Build history of the part. All positions in model axes, mm. A direction names the side the tool comes from. Round coordinates to 2 decimals unless told otherwise and drop trailing zeros. Write each loop counter-clockwise with the first axis right and the second up, starting at its lowest first coordinate (ties: lowest second). Pieces come first, ordered by that corner, then holes. Notation, with made-up numbers: M 57.25,-13.75 L 65.25,-13.75 A7 ccw 65.25,-0.75 Z; hole C -13.5,73 d8. An arc over 180 degrees is marked long. Use a Markdown table: item, result.
from build123d import *

# Parameters (mm, degrees)
SZKIC1_W                    = 115
SZKIC1_H                    = 56
DODANIE_WYCI_GNI_CIE1_DEPTH = 33
SZKIC2_R                    = 5.5
DODANIE_WYCI_GNI_CIE2_DEPTH = 22
DODANIE_WYCI_GNI_CIE3_DEPTH = 15


with BuildPart() as part:
    # Szkic1 → Dodanie-wyciągnięcie1 (new body)
    with BuildSketch(Plane(origin=(0, 0, 0), x_dir=(1, 0, 0), z_dir=(0, 1, 0))):
        with Locations((57.5, 28)):
            Rectangle(SZKIC1_W, SZKIC1_H)
    extrude(amount=DODANIE_WYCI_GNI_CIE1_DEPTH)

    # Szkic2 → Dodanie-wyciągnięcie2 (add)
    with BuildSketch(Plane(origin=(115, 0, 0), x_dir=(0, 0, -1), z_dir=(1, 0, 0))):
        with Locations((28, 16.5)):
            Circle(SZKIC2_R)
    extrude(amount=DODANIE_WYCI_GNI_CIE2_DEPTH)

    # Szkic3 → Dodanie-wyciągnięcie3 (add)
    with BuildSketch(Plane.ZY):
        Polygon((-34, 16.5), (-34, 12), (-22, 12), (-22, 16.5), (-22, 21), (-34, 21), align=None)
    extrude(amount=DODANIE_WYCI_GNI_CIE3_DEPTH)


solid = part.part
Q1. Cut at A-A on y = 16.5. Give the cut face in (x, z), and give its area (3 significant figures).
Response values:
| item | result |
|---|---|
| outline | M -15,-34 L 0,-34 L 0,-56 L 115,-56 L 115,-33.5 L 137,-33.5 L 137,-22.5 L 115,-22.5 L 115,0 L 0,0 L 0,-22 L -15,-22 Z |
| area | 6,860 mm2 |
Q2. Which spindle directions (+Z, -Z, +X, -X, +Y, -Y) get a long thin tool onto all of the face, cutting with end or side? Do faces 1 (the cylindrical face through (125.8, 13.2, -23.6)), 2 (the flat face through (-7, 21, -28)), 3 (the flat face through (-7, 17, -34)), 4 (the flat face through (-7, 12, -28)), 5 (the flat face through (-7, 16, -22)). Say none if no direction does.
Response values:
| item | result |
|---|---|
| face 1 | +X |
| face 2 | +Z, -Z, -X, +Y |
| face 3 | -Z, -X, +Y, -Y |
| face 4 | +Z, -Z, -X, -Y |
| face 5 | +Z, -X, +Y, -Y |
Q3. Cut at B-B on z = -28. Give the cut face in (x, y), and give its area (3 significant figures).
Response values:
| item | result |
|---|---|
| outline | M -15,12 L 0,12 L 0,0 L 115,0 L 115,11 L 137,11 L 137,22 L 115,22 L 115,33 L 0,33 L 0,21 L -15,21 Z |
| area | 4,170 mm2 |
Q4. Cut at C-C on y = 30. Give the cut face in (x, z), and give its area (3 significant figures).
Response values:
| item | result |
|---|---|
| outline | M 0,-56 L 115,-56 L 115,0 L 0,0 Z |
| area | 6,440 mm2 |
Q5. Drop flat-ended pins along their axis: P1, Ø3.5, axis at x = -4, z = -29, coming from the +Y side; P2, Ø8, axis at x = 101, y = 14, coming from the +Z side; P3, Ø2.5, axis at x = -5, y = 15, coming from the +Z side; P4, Ø9.5, axis at x = -10, z = -26.5, coming from the -Y side. Give the stop position or say it passes through.
Response values:
| item | result |
|---|---|
| P1 | stops at y = 21 |
| P2 | stops at z = 0 |
| P3 | stops at z = -22 |
| P4 | stops at y = 12 |
Q6. Drill centre lines: L1, parallel to X at y = 9.5, z = -6.5; L2, parallel to Y at x = 122, z = -28. Where is each one in solid material? Low to high.
Response values:
| item | result |
|---|---|
| L1 | x = 0 to 115 |
| L2 | y = 11 to 22 |
Q7. Cut at D-D on z = -12.5. Give the cut face in (x, y).
Response values:
| item | result |
|---|---|
| outline | M 0,0 L 115,0 L 115,33 L 0,33 Z |
